from build123d import *

# Parameters (mm, degrees)
BOSS_EXTRUDE1_DEPTH = 20
CUT_EXTRUDE1_REACH  = 64.285
SKETCH3_R           = 2.5


with BuildPart() as part:
    # Sketch2 → Boss-Extrude1 (new body)
    with BuildSketch(Plane(origin=(0, 0, 0), x_dir=(1, 0, 0), z_dir=(0, 1, 0))):
        with BuildLine():
            Line((-24.6, 28.345199184), (-24.6, 8))
            ThreePointArc((-24.6, 8), (-25.185786438, 6.585786438), (-26.6, 6))
            Line((-26.6, 6), (-45, 6))
            Line((-45, 6), (-45, -4))
            ThreePointArc((-45, -4), (-44.414213562, -5.414213562), (-43, -6))
            Line((-43, -6), (43.8, -6))
            ThreePointArc((43.8, -6), (45.214213562, -5.414213562), (45.8, -4))
            Line((45.8, -4), (45.8, 6))
            Line((45.8, 6), (27.4, 6))
            ThreePointArc((27.4, 6), (25.985786438, 6.585786438), (25.4, 8))
            Line((25.4, 8), (25.4, 29.172494416))
            ThreePointArc((25.4, 29.172494416), (24.133143915, 31.033273823), (21.9375, 30.536713515))
            ThreePointArc((21.9375, 30.536713515), (0.539453133, 21.004850554), (-21.1875, 29.761124235))
            ThreePointArc((-21.1875, 29.761124235), (-23.366485486, 30.192494504), (-24.6, 28.345199184))
        make_face()
    extrude(amount=BOSS_EXTRUDE1_DEPTH)

    # Sketch3 → Cut-Extrude1 (cut, up to next)
    with BuildSketch(Plane.XY.offset(6), mode=Mode.PRIVATE) as cut_extrude1_sk1:
        with Locations((-36.4, 10)):
            Circle(SKETCH3_R)
    cut_extrude1_tool1 = extrude(cut_extrude1_sk1.sketch, amount=-CUT_EXTRUDE1_REACH, mode=Mode.PRIVATE) & part.part
    # Sketch3 → Cut-Extrude1 (cut, up to next)
    with BuildSketch(Plane.XY.offset(6), mode=Mode.PRIVATE) as cut_extrude1_sk2:
        with Locations((37.2, 10)):
            Circle(SKETCH3_R)
    cut_extrude1_tool2 = extrude(cut_extrude1_sk2.sketch, amount=-CUT_EXTRUDE1_REACH, mode=Mode.PRIVATE) & part.part
    add(cut_extrude1_tool1.solids().sort_by_distance((-36.4, 10, 6))[0], mode=Mode.SUBTRACT)
    add(cut_extrude1_tool2.solids().sort_by_distance((37.2, 10, 6))[0], mode=Mode.SUBTRACT)


solid = part.part
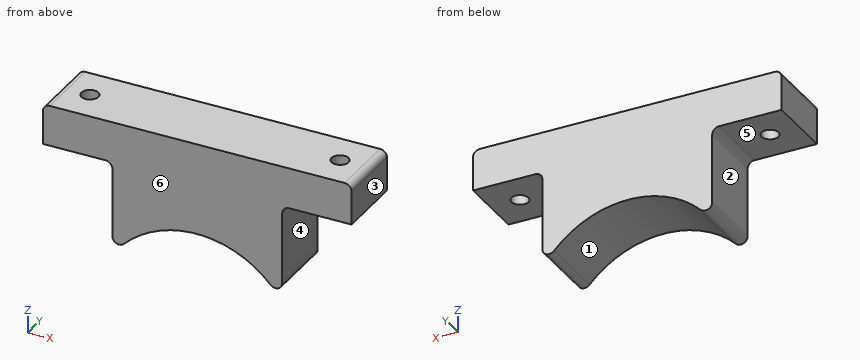
Work out the finished part from the listing and answer in its coordinate system (mm). Face numbers are marked on the shaded views. A direction names the side the tool comes from. Coordinates: 2 decimals unless noted, no trailing zeros. Write each loop counter-clockwise with the first axis right and the second up, starting at its lowest first coordinate (ties: lowest second). Pieces come first, ordered by that corner, then holes. Notation, with made-up numbers: M 52,37.25 L 110,37.25 A22 ccw 110,46.25 Z; hole C 53,67.5 d2. An arc over 180 degrees is marked long. Answer as CSV lines item,"result". Start each with the question number.
Item 1: Flat-ended cylindrical pins translate along their axes: P1, Ø4, axis at x = -36.4, y = 10, coming from the +Z side; P2, Ø4, axis at x = 9, y = 3.5, coming from the -Z side; P3, Ø6.5, axis at x = 37.2, y = 10, coming from the -Z side; P4, Ø1, axis at y = 12, z = -25, coming from the +X side. Find the tip coordinate at first contact, or state that the pin passes through.
Item 2: Section B-B on y = 11 is taken. Write down the section's boundary in (x, z), and give its area (3 significant figures).
Item 3: Section C-C on z = -4 is taken. Write down the section's boundary in (x, y).
Item 4: Determine the mould class of the marked faces 1, 2 and 3 for opening direction X: released by +X, released by -X, zero draft, split by the parting line, or undercut.
Item 5: Consider L1, parallel to Y at x = -36.4, z = 1; L2, parallel to X at y = 11.5, z = 2; L3, parallel to Z at x = -34, y = 6.5. Determine where each line is inside the solid, lowest interval first.
Item 6: Section D-D on z = -23.5 is taken. Write down the section's boundary in (x, y).
Item 7: A tool of negligible diameter and unlimited length cuts with its end or side. For the marked faces 4, 5 and 6, from which of +Z, -Z, +X, -X, +Y, -Y can it reach the whole face along a straight path? Write none if from no direction.
Item 8: Section A-A on x = 37.2 is taken. Write down the section's boundary in (y, z), and give its area (3 significant figures).
Checks:
1,P1,"passes through"
1,P2,"stops at z = -23.09"
1,P3,"stops at z = -6"
1,P4,"stops at x = 25.4"
2,outline,"M -45,-6 L -38.69,-6 L -38.69,6 L -43,6 A2 ccw -45,4 Z; M -34.11,-6 L -26.6,-6 A2 cw -24.6,-8 L -24.6,-28.35 A2 ccw -21.19,-29.76 A30 cw 21.94,-30.54 A2 ccw 25.4,-29.17 L 25.4,-8 A2 cw 27.4,-6 L 34.91,-6 L 34.91,6 L -34.11,6 Z; M 39.49,-6 L 45.8,-6 L 45.8,4 A2 ccw 43.8,6 L 39.49,6 Z"
2,area,"1,920 mm²"
3,outline,"M -45,0 L 45.8,0 L 45.8,20 L -45,20 Z; hole C -36.4,10 d5; hole C 37.2,10 d5"
4,face 1,"undercut"
4,face 2,"released by -X"
4,face 3,"released by +X"
5,L1,"y = 0 to 7.5, 12.5 to 20"
5,L2,"x = -45 to -38.4, -34.4 to 35.2, 39.2 to 45.8"
5,L3,"z = -6 to 6"
6,outline,"M -24.6,0 L -11.99,0 L -11.99,20 L -24.6,20 Z; M 11.99,0 L 25.4,0 L 25.4,20 L 11.99,20 Z"
7,face 4,"-Z, +X, +Y, -Y"
7,face 5,"-Z, -X, +Y, -Y"
7,face 6,"+Z, -Z, +X, -X, -Y"
8,outline,"M 0,-6 L 7.5,-6 L 7.5,6 L 0,6 Z; M 12.5,-6 L 20,-6 L 20,6 L 12.5,6 Z"
8,area,"180 mm²"
